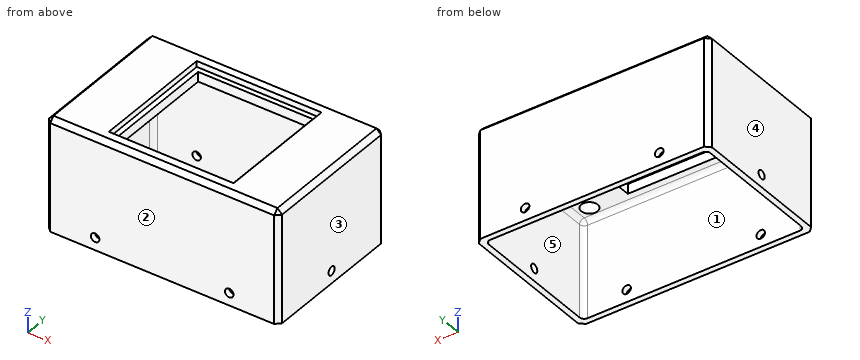
```python
from build123d import *

# Parameters (mm, degrees)
ESQUISSE1_W                     = 60
ESQUISSE1_H                     = 38
BASE_DEPTH                      = 4
ESQUISSE2_W                     = 29.5
ESQUISSE2_H                     = 29
SCREEN_DEPTH                    = 4
ESQUISSE5_R                     = 2.1
INSERTS_M3_DEPTH                = 3
ESQUISSE6_W                     = 60
ESQUISSE6_H                     = 38
ESQUISSE6_W_2                   = 57
ESQUISSE6_H_2                   = 35
WALLS_DEPTH                     = 25
CHANFREIN_EXT_SIZE              = 1.2
FILLET_INT_R                    = 1.2
ESQUISSE7_R                     = 1.1
PASSAGE_VIS_HORIZONTAL_DEPTH    = 68.720011813
ESQUISSE9_R                     = 1.1
PASSAGE_VIS_VERTICAL_DEPTH      = 55.488530903
ESQUISSE11_W                    = 32.1
ESQUISSE11_H                    = 31.6
EMPLACEMENT_VERRE_32_5_32_DEPTH = 1.5


with BuildPart() as part:
    # Esquisse1 → BASE (new body)
    with BuildSketch(Plane.XY):
        Rectangle(ESQUISSE1_W, ESQUISSE1_H)
    extrude(amount=BASE_DEPTH)

    # Esquisse2 → Screen (cut)
    with BuildSketch(Plane.XY.offset(4)):
        with Locations((0.05, 0)):
            Rectangle(ESQUISSE2_W, ESQUISSE2_H)
    extrude(amount=-SCREEN_DEPTH, mode=Mode.SUBTRACT)

    # Esquisse5 → Inserts_M3 (cut)
    with BuildSketch(Plane(origin=(0, 0, 0), x_dir=(-1, 0, 0), z_dir=(0, 0, -1))):
        with Locations((-24.3, 14)):
            Circle(ESQUISSE5_R)
        with Locations(Location((-24.3, -14, 0), (0, 0, 180))):
            Circle(ESQUISSE5_R)
        with Locations((18.6, -14)):
            Circle(ESQUISSE5_R)
        with Locations(Location((18.6, 14, 0), (0, 0, 180))):
            Circle(ESQUISSE5_R)
    extrude(amount=-INSERTS_M3_DEPTH, mode=Mode.SUBTRACT)

    # Esquisse6 → Walls (add)
    with BuildSketch(Plane(origin=(0, 0, 0), x_dir=(-1, 0, 0), z_dir=(0, 0, -1))):
        Rectangle(ESQUISSE6_W, ESQUISSE6_H)
        Rectangle(ESQUISSE6_W_2, ESQUISSE6_H_2, mode=Mode.SUBTRACT)
    extrude(amount=WALLS_DEPTH)

    # Chanfrein_EXT
    chanfrein_ext_edges = [part.edges().sort_by_distance(p)[0] for p in [
        (30, 0, 4),
        (0, 19, 4),
        (-30, 0, 4),
        (-30, 19, -10.5),
        (30, 19, -10.5),
        (30, -19, -10.5),
        (-30, -19, -10.5),
        (0, -19, 4),
    ]]
    chamfer(chanfrein_ext_edges, length=CHANFREIN_EXT_SIZE)

    # Fillet_INT
    fillet_int_edges = [part.edges().sort_by_distance(p)[0] for p in [
        (0, 17.5, 0),
        (28.5, 0, 0),
        (0, -17.5, 0),
        (-28.5, 0, 0),
        (28.5, 17.5, -12.5),
        (28.5, -17.5, -12.5),
        (-28.5, -17.5, -12.5),
        (-28.5, 17.5, -12.5),
    ]]
    fillet(fillet_int_edges, radius=FILLET_INT_R)

    # Esquisse7 → Passage_Vis_Horizontal (cut, through all)
    with BuildSketch(Plane(origin=(30, 0, 0), x_dir=(0, 0, -1), z_dir=(1, 0, 0))):
        with Locations(Location((21.8, 0, 0), (0, 0, 90))):
            Circle(ESQUISSE7_R)
    extrude(amount=-PASSAGE_VIS_HORIZONTAL_DEPTH, mode=Mode.SUBTRACT)

    # Esquisse9 → Passage_Vis_Vertical (cut, through all)
    with BuildSketch(Plane(origin=(0, 19, 0), x_dir=(1, 0, 0), z_dir=(0, 1, 0))):
        with Locations(Location((-17.25, 21.8, 0), (0, 0, 180))):
            Circle(ESQUISSE9_R)
        with Locations(Location((17.25, 21.8, 0), (0, 0, 180))):
            Circle(ESQUISSE9_R)
    extrude(amount=-PASSAGE_VIS_VERTICAL_DEPTH, mode=Mode.SUBTRACT)

    # Esquisse11 → Emplacement Verre 32.5*32 (cut)
    with BuildSketch(Plane.XY.offset(4)):
        with Locations((0.05, 0)):
            Rectangle(ESQUISSE11_W, ESQUISSE11_H)
    extrude(amount=-EMPLACEMENT_VERRE_32_5_32_DEPTH, mode=Mode.SUBTRACT)


solid = part.part
```
Input: part model. Units: mm. Frame: model coordinates. Face numbers are marked on the shaded views. A direction names the side the tool comes from. Coordinates: 2 decimals unless noted, no trailing zeros. Loops run counter-clockwise (first coordinate to the right, second up) from the corner with the lowest first, then second, coordinate; pieces in that order, holes last. Notation, with made-up numbers: M -1.5,89 L 37.5,89 A21 ccw 37.5,112 Z; hole C 7.5,20 d1. An arc over 180 degrees is marked long. Answer in a Markdown table with one row per item.
1. Section C-C, the plane y = 0. Output: boundary loops of the cut face in (x, z).
Response:
| item | result |
|---|---|
| outline | M -30,-25 L -28.5,-25 L -28.5,-22.9 L -30,-22.9 Z; M -30,-20.7 L -28.5,-20.7 L -28.5,-1.2 A1.2 cw -27.3,0 L -14.7,0 L -14.7,2.5 L -16,2.5 L -16,4 L -28.8,4 L -30,2.8 Z; M 14.8,0 L 27.3,0 A1.2 cw 28.5,-1.2 L 28.5,-20.7 L 30,-20.7 L 30,2.8 L 28.8,4 L 16.1,4 L 16.1,2.5 L 14.8,2.5 Z; M 28.5,-25 L 30,-25 L 30,-22.9 L 28.5,-22.9 Z |
2. Section A-A, the plane y = -7.5. Output: boundary loops of the cut face in (x, z).
Response:
| item | result |
|---|---|
| outline | M -30,-25 L -28.5,-25 L -28.5,-1.2 A1.2 cw -27.3,0 L -14.7,0 L -14.7,2.5 L -16,2.5 L -16,4 L -28.8,4 L -30,2.8 Z; M 14.8,0 L 27.3,0 A1.2 cw 28.5,-1.2 L 28.5,-25 L 30,-25 L 30,2.8 L 28.8,4 L 16.1,4 L 16.1,2.5 L 14.8,2.5 Z |
3. Draft query along X for the marked faces 3, 4 and 5. Return one class per face: pulls with the +X half, pulls with the -X half, needs draft (parallel to the pull), parting line crosses it, or undercut.
Response:
| item | result |
|---|---|
| face 3 | pulls with the +X half |
| face 4 | pulls with the -X half |
| face 5 | undercut |
4. Reachability of the marked faces 1 and 2 from +Z, -Z, +X, -X, +Y, -Y: full face, straight path, thin tool, end or side. Return the list, or none.
Response:
| item | result |
|---|---|
| face 1 | -Z |
| face 2 | +Z, -Z, +X, -X, -Y |
5. Material intervals for line 1 (Y direction, x = 24.3, z = 1.05); line 2 (X direction, y = 6.5, z = -7.75); line 3 (Y direction, x = -25.5, z = -8.5), sorted ascending.
Response:
| item | result |
|---|---|
| line 1 | y = -19 to -16.1, -11.9 to 11.9, 16.1 to 19 |
| line 2 | x = -30 to -28.5, 28.5 to 30 |
| line 3 | y = -19 to -17.5, 17.5 to 19 |
6. Section D-D, the plane z = -16.5. Output: boundary loops of the cut face in (x, y), then the cut area to 3 significant figures.
Response:
| item | result |
|---|---|
| outline | M -30,-17.8 L -28.8,-19 L 28.8,-19 L 30,-17.8 L 30,17.8 L 28.8,19 L -28.8,19 L -30,17.8 Z; hole M -28.5,-16.3 A1.2 ccw -27.3,-17.5 L 27.3,-17.5 A1.2 ccw 28.5,-16.3 L 28.5,16.3 A1.2 ccw 27.3,17.5 L -27.3,17.5 A1.2 ccw -28.5,16.3 Z |
| area | 283 mm2 |
7. Section B-B, the plane x = -12. Output: boundary loops of the cut face in (y, z).
Response:
| item | result |
|---|---|
| outline | M -19,-25 L -17.5,-25 L -17.5,-1.2 A1.2 cw -16.3,0 L -14.5,0 L -14.5,2.5 L -15.8,2.5 L -15.8,4 L -17.8,4 L -19,2.8 Z; M 14.5,0 L 16.3,0 A1.2 cw 17.5,-1.2 L 17.5,-25 L 19,-25 L 19,2.8 L 17.8,4 L 15.8,4 L 15.8,2.5 L 14.5,2.5 Z |
8. First-contact query: pin 1 (1.2 mm diameter, centred on y = 2, z = 3.5, fed in from +X); pin 2 (1.3 mm diameter, centred on x = -18.5, y = -14.5, fed in from -Z). Flat tips, straight axial feed; report the tip coordinate or a pass-through.
Response:
| item | result |
|---|---|
| pin 1 | stops at x = 29.9 |
| pin 2 | stops at z = 3 |
